Input: dimensioned drawing with shaded views. Units: mm. Origin: part minimum x, y, z. A direction names the side the tool comes from. Round coordinates to 2 decimals unless told otherwise and drop trailing zeros. Write each loop counter-clockwise with the first axis right and the second up, starting at its lowest first coordinate (ties: lowest second). Pieces come first, ordered by that corner, then holes. Notation, with made-up numbers: M 16.25,54 L 42.25,54 A15 cw 42.25,63 Z; hole C 78,-32.5 d6. An arc over 180 degrees is marked long. Answer as CSV lines item,"result". Start each with the question number.
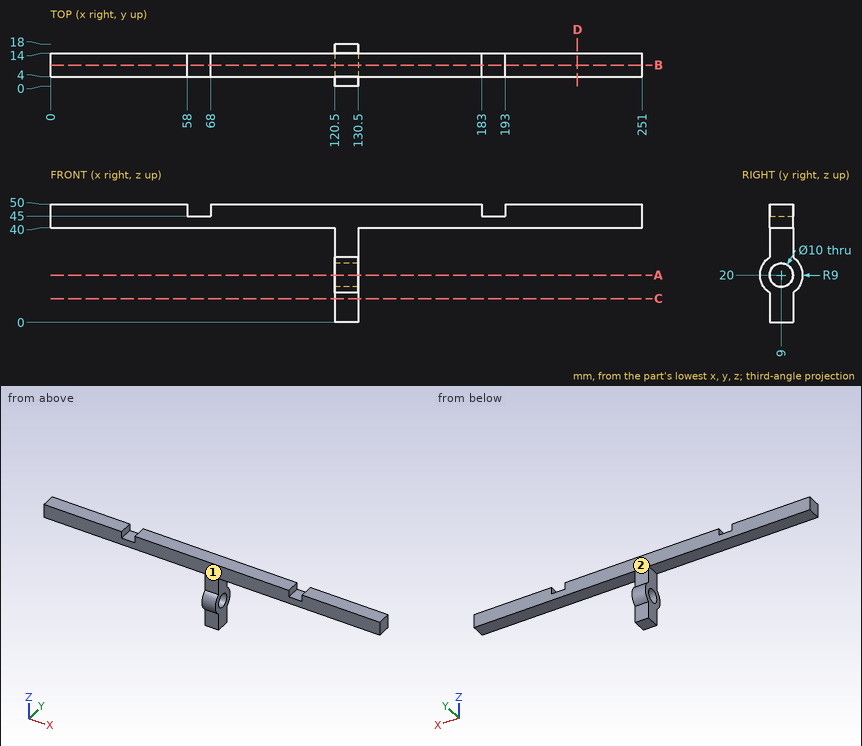
Item 1: Cut plane B-B, the plane y = 9. Return loops of the section in (x, z).
Item 2: Cut plane D-D, the plane x = 223.5. Return loops of the section in (y, z), plus the area to 3 significant figures.
Item 3: Cut plane A-A, the plane z = 20. Return loops of the section in (x, y).
Item 4: Cut plane C-C, the plane z = 10. Return loops of the section in (x, y).
Item 5: Pin query (flat end, axial travel): pin 1 Ø10 at (x, z) = (222.5, 42.5) entering from -Y; pin 2 Ø3 at (x, z) = (124, 4.5) entering from +Y; pin 3 Ø3 at (y, z) = (7, 23.5) entering from +X. Return the tip coordinate at first contact, or that it passes through.
Item 6: Access query for the marked faces 1 and 2. Directions: +Z, -Z, +X, -X, +Y, -Y. A direction counts if a zero-diameter tool reaches every point of the face in a straight line with its end or side. Return the directions, or none.
Item 7: Line query: line 1 (Y direction, x = 125, z = 20); line 2 (Z direction, x = 127.25, y = 9); line 3 (X direction, y = 13.75, z = 6). Output: solid intervals per line, ascending. Write a range as [from, to].
Results list:
1,outline,"M 0,40 L 120.5,40 L 120.5,25 L 130.5,25 L 130.5,40 L 251,40 L 251,50 L 193,50 L 193,45 L 183,45 L 183,50 L 68,50 L 68,45 L 58,45 L 58,50 L 0,50 Z; M 120.5,0 L 130.5,0 L 130.5,15 L 120.5,15 Z"
2,outline,"M 4,40 L 14,40 L 14,50 L 4,50 Z"
2,area,"100 mm²"
3,outline,"M 120.5,0 L 130.5,0 L 130.5,4 L 120.5,4 Z; M 120.5,14 L 130.5,14 L 130.5,18 L 120.5,18 Z"
4,outline,"M 120.5,4 L 130.5,4 L 130.5,14 L 120.5,14 Z"
5,pin 1,"y = 4"
5,pin 2,"y = 14"
5,pin 3,"x = 130.5"
6,face 1,"+Z, +X, -X, -Y"
6,face 2,"+Z, +X, -X, +Y"
7,line 1,"[0, 4], [14, 18]"
7,line 2,"[0, 15], [25, 50]"
7,line 3,"[120.5, 130.5]"
